Design review of the part shown in the three views and the two pictorial views. Dimensions are in mm from the part's minimum x, y and z. A direction names the side the tool comes from. Coordinates: 2 decimals unless noted, no trailing zeros. Loops run counter-clockwise (first coordinate to the right, second up) from the corner with the lowest first, then second, coordinate; pieces in that order, holes last. Notation, with made-up numbers: (52, 26) - (83, 26) arc R29 ccw to (83, 61) - close; hole circle Ø10 at (87.25, -4.75). An arc over 180 degrees is marked (long way). One line per item, written item: value. Start each with the question number.
1. Take a section at C-C, the plane x = 46.5. State the section outline as (y, z) points, and give its area (3 significant figures).
2. For the marked faces 4 and 5, list the 3-axis set-ups (+Z, -Z, +X, -X, +Y, -Y) from which the entire face can be reached by the end or side of a thin tool; tool diameter is ignored.
3. Take a section at A-A, the plane z = 77.5. Count the separate pieces of the cut face and the enclosed holes in it, and give its area (3 significant figures).
4. The part is to be moulded in two halves that separate along X. For the marked faces 1, 2 and 3, say which applies: released by +X, released by -X, zero draft, split by the parting line, or undercut.
5. Take a section at D-D, the plane z = 9. State the section outline as (x, y) points.
6. To check wall thickness, follow line 1 (Z direction, x = 67.5, y = 47.5); line 2 (X direction, y = 20, z = 70) (1 decimal); line 3 (Y direction, x = 69.5, z = 21). State the ranges of each line that lie inside material, in increasing order. Write a range as from..to.
7. Take a section at B-B, the plane y = 15.5. State the section outline as (x, z) points (1 decimal).
8. Insertion check: pin 1 (12 mm diameter, centred on y = 16.5, z = 27.5, fed in from -X); pin 2 (2 mm diameter, centred on y = 28, z = 83.5, fed in from -X); pin 3 (12 mm diameter, centred on y = 54, z = 38.5, fed in from -X); pin 4 (12 mm diameter, centred on x = 45, y = 50, fed in from +Z). Each pin has a flat end and moves straight along its axis. Give the tip position at first contact, or say it passes through.
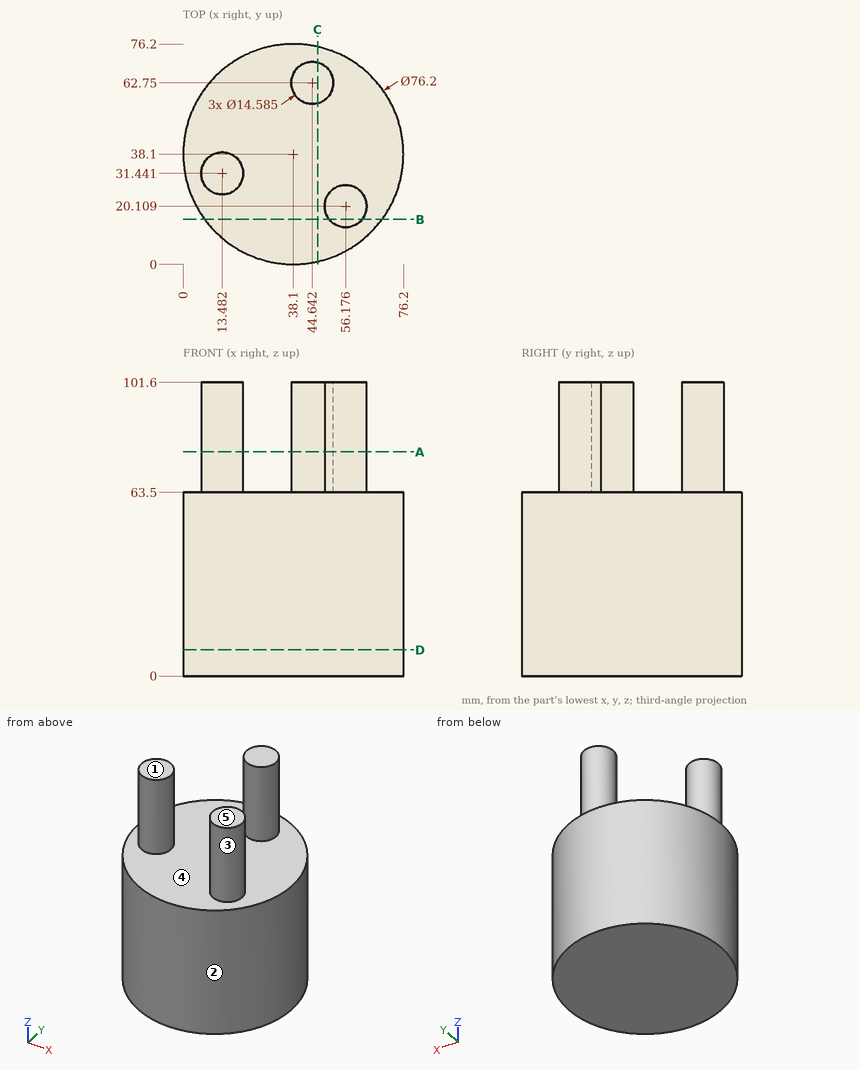
Solutions:
1. outline: (0.94, 0) - (75.26, 0) - (75.26, 63.5) - (69.8, 63.5) - (69.8, 101.6) - (55.7, 101.6) - (55.7, 63.5) - (0.94, 63.5) - close
1. area: 5,260 mm2
2. face 4: +Z
2. face 5: +Z, +X, -X, +Y, -Y
3. separate pieces: 3
3. enclosed holes: 0
3. area: 501 mm2
4. face 1: zero draft
4. face 2: split by the parting line
4. face 3: undercut
5. outline: circle Ø76.2 at (38.1, 38.1)
6. line 1: 0..63.5
6. line 2: 48.9..63.5
6. line 3: 16.52..59.68
7. outline: (7.4, 0) - (68.8, 0) - (68.8, 63.5) - (61.8, 63.5) - (61.8, 101.6) - (50.5, 101.6) - (50.5, 63.5) - (7.4, 63.5) - close
8. pin 1: x = 3.34
8. pin 2: x = 6.61
8. pin 3: x = 1.31
8. pin 4: z = 101.6
